Autodesk Inventor part; units mm, degrees
ref_plane "Work Plane1" through (0, 0, -3) normal (0, 0, 1) x (1, 0, 0)
ref_plane "YZ Plane" through (0, 0, 0) normal (1, 0, 0) x (0, 1, 0)
ref_plane "XZ Plane" through (0, 0, 0) normal (0, 1, 0) x (-1, 0, 0)
ref_plane "Work Plane1" through (0, 0, -3) normal (0, 0, 1) x (1, 0, 0)
sketch "Sketch1" plane through (0, 0, -3) normal (0, 0, 1) x (1, 0, 0)
  circle A0 centre (0, 0) radius 2.75
extrude "Extrusion3" add sketch "Sketch1" along normal blind 3
fillet "Fillet1" radius 0.1 2 edges at (-2.75, 0, -3) (-2.75, 0, 0)
sketch "Sketch2" plane through (0, 0, -3) normal (0, 0, 1) x (1, 0, 0)
  line L0 (-0.7217, 1.25) -> (0.7217, 1.25)
  line L1 (0.7217, -1.25) -> (-0.7217, -1.25)
  line L2 (-0.7217, -1.25) -> (-1.4434, 0)
  line L3 (0.7217, 1.25) -> (1.4434, 0)
  line L4 (-1.4434, 0) -> (-0.7217, 1.25)
  line L5 (1.4434, 0) -> (0.7217, -1.25)
extrude "Extrusion2" cut sketch "Sketch2" along normal blind 3
sketch "Sketch3" plane through (0, 0, 0) normal (0, 0, 1) x (1, 0, 0)
  circle A0 centre (0, 0) radius 1.5
extrude "Extrusion1" add sketch "Sketch3" along normal blind 18
chamfer "Chamfer1" distance 0.2 angle 45 1 edges at (-1.5, 0, 18)
properties part number "DIN 912 M3 8 mm" material "Stainless Steel"
Geometry: final body of the model. Coordinates: model frame, mm. A direction names the side the tool comes from. Round coordinates to 2 decimals unless told otherwise and drop trailing zeros. Loops run counter-clockwise (first coordinate to the right, second up) from the corner with the lowest first, then second, coordinate; pieces in that order, holes last. Notation, with made-up numbers: M 87,71 L 118,71 A18 cw 118,96 Z; hole C 8,62.25 d1. An arc over 180 degrees is marked long. Put each result on its own line as item: value. Start each with the question number.
(1) Contact query for flat-ended pins moving along their axis: pin 1 Ø3 at (x, z) = (2, 13.5) entering from +Y; pin 2 Ø3 at (y, z) = (-2, 0) entering from +X. Output: stop coordinate, or through.
(2) Draft query along Y for faces 1 (the face through (0, -2, 0)), 2 (the face through (0, 0, 0)), 3 (the face through (-0.596, 2.685, -1.52)). Return one class per face: +Y half, -Y half, draft (parallel to the pull), parting line (faces both ways), or undercut.
(3) Set-up query: faces 4 (the face through (0, 0, 18)), 5 (the face through (-1.088, 0.616, -1.521)), 6 (the face through (-1.5, -0.07, 8.78)). Return all of +Z, -Z, +X, -X, +Y, -Y with unobstructed straight access to the full face (end or side cutting, diameter ignored); none if empty.
(4) Section query A-A (x = 0). Return loops of the section in (y, z), then the cut area to 3 significant figures.
(5) Section query B-B (z = 6.5). Return loops of the section in (x, y), then the cut area to 3 significant figures.
(6) Material intervals for line 1 along Z through (x, y) = (0.4, -1.6); line 2 along Z through (x, y) = (0.05, -0.8); line 3 along Y through (x, z) = (0.4, 7), sorted ascending. Write a range as [from, to].
Findings below:
1. pin 1: stops at y = 1.41
1. pin 2: stops at x = 2.7
2. face 1: draft
2. face 2: undercut
2. face 3: parting line
3. face 4: +Z, +X, -X, +Y, -Y
3. face 5: -Z
3. face 6: +Z
4. outline: M -2.75,-2.9 A0.1 ccw -2.65,-3 L -1.25,-3 L -1.25,0 L 1.25,0 L 1.25,-3 L 2.65,-3 A0.1 ccw 2.75,-2.9 L 2.75,-0.1 A0.1 ccw 2.65,0 L 1.5,0 L 1.5,17.8 L 1.3,18 L -1.3,18 L -1.5,17.8 L -1.5,0 L -2.65,0 A0.1 ccw -2.75,-0.1 Z
4. area: 63.0 mm2
5. outline: C 0,0 d3
5. area: 7.07 mm2
6. line 1: z = [-3, 0]
6. line 2: z = [0, 18]
6. line 3: y = [-1.45, 1.45]
